For this review, take the finished solid that the model builds, in its own axes (mm). A direction names the side the tool comes from. Coordinates: 2 decimals unless noted, no trailing zeros. Loops run counter-clockwise (first coordinate to the right, second up) from the corner with the lowest first, then second, coordinate; pieces in that order, holes last. Notation, with made-up numbers: (6, 55) - (50, 55) arc R21 cw to (50, 85) - close; hole circle Ø2 at (-26.5, 89). An arc over 180 degrees is marked (long way). Use one line per item in the form item = value. Start each with the question number.
1. Machinability: for faces 1 (the face through (55, 40, 115)), 2 (the face through (-77.5, -1, 2)), 3 (the face through (75, -20, 102.5)), 4 (the face through (-1, -1, -112.5)), which of the approach directions +Z, -Z, +X, -X, +Y, -Y give a long, thin tool a straight path to every point of the face, cutting with its end or side? Answer none if there is none.
2. Add section C-C on y = 3. Give the boundary of the cut face in (x, z), and give its area (4 significant figures).
3. To check wall thickness, follow probe 1 along Z at (x, y) = (15.5, -9.5); probe 2 along Y at (x, z) = (56, 80.5); probe 3 along Z at (x, y) = (0, 51.45). State the ranges of each line that lie inside material, in increasing order.
4. For pin 1 Ø21 at (x, z) = (13, 53) entering from +Y, flat-tipped, find the tip position at first contact; note if it passes through.
5. Add section B-B on z = 53.5. Give the boundary of the cut face in (x, y), and give its area (3 significant figures).
6. Draft analysis for pull direction Z (two halves, no side actions). For faces 5 (the face through (1, -50, -62)), 6 (the face through (62.5, 25, 115)), 7 (the face through (1, -1, 112.5)), 8 (the face through (-1, -1, -117.5)), state which applies: +Z half, -Z half, draft (parallel to the pull), parting line (faces both ways), or undercut.
7. Add section A-A on x = 55.5. Give the boundary of the cut face in (y, z).
8. Add section D-D on x = 29. Give the boundary of the cut face in (y, z), and give its area (3 significant figures).
Autodesk Inventor part; units mm, degrees
ref_plane "YZ Plane" through (0, 0, 0) normal (1, 0, 0) x (0, 1, 0)
ref_plane "XZ Plane" through (0, 0, 0) normal (0, 1, 0) x (-1, 0, 0)
ref_plane "XY Plane" through (0, 0, 0) normal (0, 0, 1) x (1, 0, 0)
sketch "Sketch1" plane through (0, 0, 0) normal (0, 1, 0) x (-1, 0, 0)
  line L0 (-77.5, 117.5) -> (77.5, 117.5)
  line L1 (77.5, 117.5) -> (77.5, -117.5)
  line L2 (77.5, -117.5) -> (-77.5, -117.5)
  line L3 (-77.5, -117.5) -> (-77.5, 117.5)
  line L4 (-77.5, 117.5) -> (77.5, -117.5) construction
  line L5 (77.5, 117.5) -> (-77.5, -117.5) construction
  point P0 (0, 0)
  dimension "d0" = 235
  dimension "d1" = 155
extrude "Extrusion1" add sketch "Sketch1" along normal mid plane 110
shell "Shell1" thickness 5 removed faces 1 at (25.8333, 55, 39.1667)
sketch "Sketch2" plane through (-72.5, -50, -112.5) normal (0, 0, 1) x (1, 0, 0)
  line L0 (0, 0) -> (0, 105)
  line L1 (145, 105) -> (145, 0)
  line L2 (0, 105) -> (145, 105)
  line L3 (145, 105) -> (145, 100)
  line L4 (145, 100) -> (0, 100)
  line L5 (0, 100) -> (0, 105)
  point P0 (72.5, 50)
  point P1 (145, 105)
  dimension "d5" = 5
extrude "Extrusion2" add sketch "Sketch2" along normal through all
sketch "Sketch3" plane through (0, 55, 0) normal (0, 1, 0) x (1, 0, 0)
  line L0 (62.5, -87.5) -> (-7.5, -87.5)
  line L1 (-7.5, -87.5) -> (-7.5, -17.5)
  line L2 (-7.5, -17.5) -> (62.5, -17.5)
  line L3 (62.5, -17.5) -> (62.5, -87.5)
  line L4 (62.5, -87.5) -> (-7.5, -17.5) construction
  line L5 (-7.5, -87.5) -> (62.5, -17.5) construction
  line L6 (-77.5, 117.5) -> (-77.5, -117.5)
  line L7 (-77.5, -117.5) -> (77.5, -117.5)
  line L8 (77.5, 117.5) -> (-77.5, 117.5)
  circle A0 centre (0, 57.5) radius 20
  line L9 (77.5, -117.5) -> (77.5, 117.5)
  line L10 (-62.5, -102.5) -> (-22.5, -102.5)
  line L11 (-22.5, -102.5) -> (-22.5, -2.5)
  line L12 (-22.5, -2.5) -> (-62.5, -2.5)
  line L13 (-62.5, -2.5) -> (-62.5, -102.5)
  circle A1 centre (0, 57.5) radius 45 construction
  point P0 (0, 0)
  point P1 (27.5, -52.5)
  point P2 (-42.5, -52.5)
  dimension "d12" = 70
  dimension "d13" = 70
  dimension "d20" = 40
  dimension "d31" = 15
  dimension "d32" = 100
  dimension "d33" = 40
  dimension "d34" = 15
  dimension "d35" = 15
  dimension "d37" = 0
  dimension "d38" = 65
  dimension "d40" = 0
  dimension "d41" = 60
  dimension "d42" = 90
sketch "Sketch4" plane through (77.5, -55, -117.5) normal (1, 0, 0) x (0, 0, -1)
  line L0 (-220, 55) -> (-180, 55)
  line L1 (-180, 55) -> (-180, 15)
  line L2 (-180, 15) -> (-220, 15)
  line L3 (-220, 15) -> (-220, 55)
  line L4 (0, 0) -> (-235, 0)
  line L5 (-235, 0) -> (-235, 110)
  point P0 (-117.5, 55)
  dimension "d23" = 40
  dimension "d24" = 40
  dimension "d25" = 15
  dimension "d26" = 15
sketch "Sketch5" plane through (-77.5, 55, 117.5) normal (0, 0, 1) x (1, 0, 0)
  line L0 (125, -15) -> (140, -15)
  line L1 (140, -15) -> (140, -45)
  line L2 (140, -45) -> (125, -45)
  line L3 (125, -45) -> (125, -15)
  line L4 (0, 0) -> (155, 0)
  line L5 (155, -110) -> (155, 0)
  point P0 (77.5, -55)
  dimension "d27" = 30
  dimension "d28" = 15
  dimension "d29" = 15
  dimension "d30" = 15
sketch "Sketch6" plane through (-72.5, -50, -112.5) normal (0, 1, 0) x (1, 0, 0)
  line L0 (0, 0) -> (145, 0) construction
  line L1 (-5, -230) -> (-5, 5) construction
  line L2 (0, 0) -> (0, -100) construction
  line L3 (0, -225) -> (0, 0)
  line L4 (145, 0) -> (145, -225)
  line L5 (0, -100) -> (145, -100)
  line L6 (145, -100) -> (145, -105) construction
  line L7 (145, -105) -> (0, -105)
  line L8 (0, -105) -> (0, -100) construction
  line L9 (0, -100) -> (0, -105)
  line L10 (145, -100) -> (145, -105)
  point P0 (72.5, -112.5)
  point P1 (0, -105)
  dimension "d44" = 100
  dimension "d45" = 5
extrude "Extrusion3" add sketch "Sketch6" along normal through all
extrude "Extrusion4" cut sketch "Sketch3" against normal blind 10 contours A0
extrude "Extrusion5" cut sketch "Sketch4" against normal blind 10
extrude "Extrusion6" cut sketch "Sketch5" against normal blind 10
extrude "Extrusion7" cut sketch "Sketch3" against normal blind 0.1 contours L0 L1 L2 L3 | L13 L12 L11 L10
properties part number "estruc_mec" material "Wood (Cherry)"
Conclusion:
q1.face_1 = +Z
q1.face_2 = +Z, -Z, -X, +Y, -Y
q1.face_3 = +X
q1.face_4 = none
q2.outline = (-77.5, -117.5) - (77.5, -117.5) - (77.5, 117.5) - (-77.5, 117.5) - close; hole (-72.5, -112.5) - (72.5, -112.5) - (72.5, -12.5) - (-72.5, -12.5) - close; hole (-72.5, -7.5) - (72.5, -7.5) - (72.5, 112.5) - (-72.5, 112.5) - close
q2.area = 4,525 mm^2
q3.probe_1 = -117.5 to -112.5, -12.5 to -7.5, 112.5 to 117.5
q3.probe_2 = -55 to -50, 50 to 54.9
q3.probe_3 = -117.5 to -77.5, -37.5 to 117.5
q4.pin_1 = 54.9
q5.outline = (-77.5, -55) - (77.5, -55) - (77.5, 55) - (62.5, 55) - (62.5, 54.9) - (-7.5, 54.9) - (-7.5, 55) - (-22.5, 55) - (-22.5, 54.9) - (-62.5, 54.9) - (-62.5, 55) - (-77.5, 55) - close; hole (-72.5, -50) - (72.5, -50) - (72.5, 50) - (-72.5, 50) - close
q5.area = 2,540 mm^2
q6.face_5 = undercut
q6.face_6 = draft
q6.face_7 = undercut
q6.face_8 = -Z half
q7.outline = (-55, -117.5) - (55, -117.5) - (55, 17.5) - (54.9, 17.5) - (54.9, 87.5) - (55, 87.5) - (55, 117.5) - (40, 117.5) - (40, 112.5) - (50, 112.5) - (50, -7.5) - (-50, -7.5) - (-50, 112.5) - (10, 112.5) - (10, 117.5) - (-55, 117.5) - close; hole (-50, -112.5) - (50, -112.5) - (50, -12.5) - (-50, -12.5) - close
q8.outline = (-55, -117.5) - (55, -117.5) - (55, 17.5) - (54.9, 17.5) - (54.9, 87.5) - (55, 87.5) - (55, 117.5) - (-55, 117.5) - close; hole (-50, -112.5) - (50, -112.5) - (50, -12.5) - (-50, -12.5) - close; hole (-50, -7.5) - (50, -7.5) - (50, 112.5) - (-50, 112.5) - close
q8.area = 3,840 mm^2
